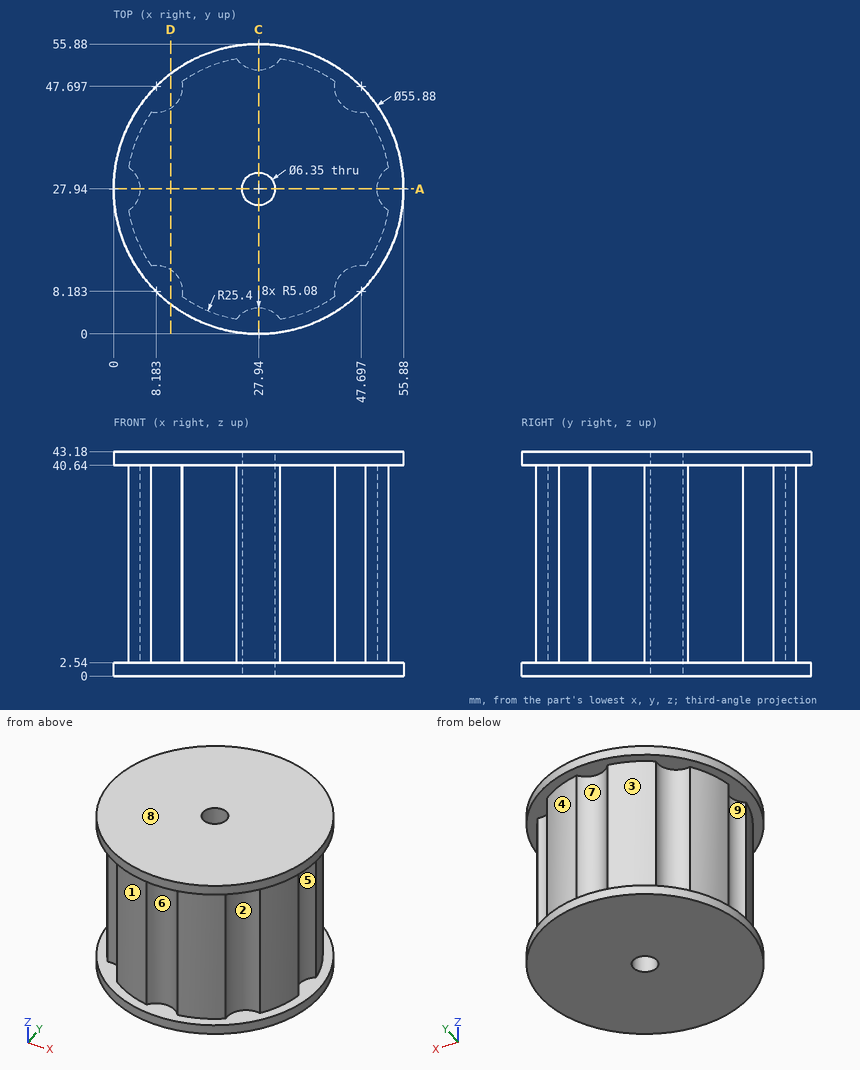
Answer from the drawing. Dimensions are ordinates in mm from the lowest x, y and z of the part. A direction names the side the tool comes from. Give positions to 0.01 mm unless a question says otherwise; leave off trailing zeros. Order: outer loops, then holes, each group sorted by start corner. A loop starts at its lowest first (then second) coordinate and runs counter-clockwise, first axis right, second up. Notation, with made-up numbers: (18.25, 22.25) -> (28.25, 22.25) arc R23 ccw to (28.25, 34.25) -> close; hole circle Ø4 at (4.25, -37). An arc over 180 degrees is marked (long way). One line per item, written item: value.
Item 1: Find section D-D, the plane x = 11. Give the vertices of the cut face in (y, z).
Answer sheet:
outline: (5.72, 0) -> (50.16, 0) -> (50.16, 2.54) -> (43.47, 2.54) -> (43.47, 40.64) -> (50.16, 40.64) -> (50.16, 43.18) -> (5.72, 43.18) -> (5.72, 40.64) -> (12.41, 40.64) -> (12.41, 2.54) -> (5.72, 2.54) -> close
Item 2: Find section A-A, the plane y = 27.94. Give the vertices of the cut face in (x, z) (1 decimal), plus the area to 3 significant figures.
Answer sheet:
outline: (0, 0) -> (24.8, 0) -> (24.8, 43.2) -> (0, 43.2) -> (0, 40.6) -> (5.1, 40.6) -> (5.1, 2.5) -> (0, 2.5) -> close; (31.1, 0) -> (55.9, 0) -> (55.9, 2.5) -> (50.8, 2.5) -> (50.8, 40.6) -> (55.9, 40.6) -> (55.9, 43.2) -> (31.1, 43.2) -> close
area: 1,750 mm²
Item 3: Flat-ended cylindrical pins translate along their axes: P1, Ø8, axis at x = 29, z = 28.5, coming from the +Y side; P2, Ø1.5, axis at x = 20, z = 36.5, coming from the +Y side; P3, Ø1.5, axis at y = 11.5, z = 30.5, coming from the +X side. Find the tip coordinate at first contact, or state that the pin passes through.
Answer sheet:
P1: y = 52.99
P2: y = 52.3
P3: x = 44.65
Item 4: A tool of negligible diameter and unlimited length cuts with its end or side. For the marked faces 1, 2, 3, 4 and 5, from which of +Z, -Z, +X, -X, +Y, -Y can it reach the whole face along a straight path? Write none if from no direction.
Answer sheet:
face 1: -X, -Y
face 2: none
face 3: -X, +Y
face 4: +X, +Y
face 5: +X
Item 5: Determine the mould class of the marked faces 6, 7, 8 and 9 for opening direction X: released by +X, released by -X, zero draft, split by the parting line, or undercut.
Answer sheet:
face 6: undercut
face 7: undercut
face 8: zero draft
face 9: released by -X
Item 6: Straight lines are drawn through the part: probe 1 along X at (y, z) = (27.94, 16.5) (1 decimal); probe 2 along Y at (x, z) = (48, 14.5) (1 decimal). For each, find the intervals that lie inside material, in ascending order.
Answer sheet:
probe 1: 5.1 to 24.8, 31.1 to 50.8
probe 2: 13.3 to 42.6
